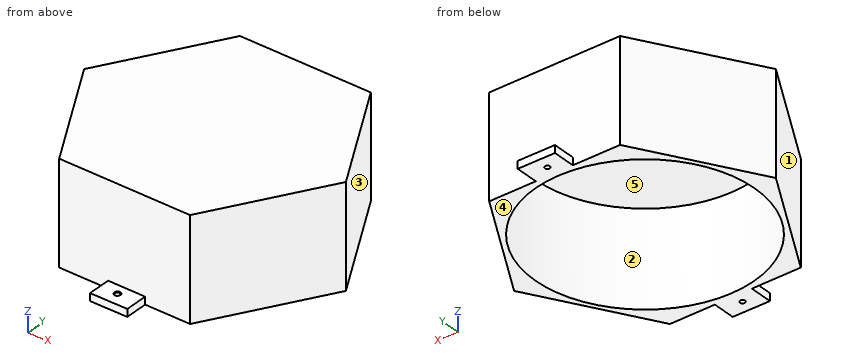
from build123d import *

# Parameters (mm, degrees)
BOSS_EXTRUDE4_DEPTH                = 40
BOSS_EXTRUDE4_DEPTH_BACK           = 1
SKETCH10_R                         = 44
CUT_EXTRUDE3_DEPTH                 = 38
SKETCH11_W                         = 15
SKETCH11_H                         = 10
BOSS_EXTRUDE5_DEPTH                = 3
M2_5X0_45_TAPPED_HOLE3_D           = 2.05
M2_5X0_45_TAPPED_HOLE3_CSINK_D     = 2.55
M2_5X0_45_TAPPED_HOLE3_CSINK_ANGLE = 90
BOSS_EXTRUDE6_DEPTH                = 41
SKETCH17_R                         = 44
CUT_EXTRUDE4_DEPTH                 = 38


with BuildPart() as part:
    # Sketch1 → Boss-Extrude4 (new body, two sides)
    with BuildSketch(Plane.XY) as boss_extrude4_sk:
        Polygon((52.078255867, 0), (26.039127933, 45.101092565), (-26.039127933, 45.101092565), (-52.078255867, 0), (-26.039127933, -45.101092565), (26.039127933, -45.101092565), align=None)
    extrude(amount=BOSS_EXTRUDE4_DEPTH)
    extrude(boss_extrude4_sk.sketch, amount=-BOSS_EXTRUDE4_DEPTH_BACK)

    # Sketch10 → Cut-Extrude3 (cut)
    with BuildSketch(Plane(origin=(0, 0, -1), x_dir=(-1, 0, 0), z_dir=(0, 0, -1))):
        Circle(SKETCH10_R)
    extrude(amount=-CUT_EXTRUDE3_DEPTH, mode=Mode.SUBTRACT)

    # Sketch11 → Boss-Extrude5 (add)
    with BuildSketch(Plane(origin=(0, 0, -1), x_dir=(-1, 0, 0), z_dir=(0, 0, -1))):
        with Locations((-0.468011799, 50.101092565)):
            Rectangle(SKETCH11_W, SKETCH11_H)
        with Locations((-0.468011799, -50.101092565)):
            Rectangle(SKETCH11_W, SKETCH11_H)
    extrude(amount=-BOSS_EXTRUDE5_DEPTH)

    # M2.5x0.45 Tapped Hole3 (through all)
    with Locations(Plane.XY.offset(2)):
        with Locations((0, 50), (0, -50)):
            CounterSinkHole(M2_5X0_45_TAPPED_HOLE3_D / 2, M2_5X0_45_TAPPED_HOLE3_CSINK_D / 2, counter_sink_angle=M2_5X0_45_TAPPED_HOLE3_CSINK_ANGLE)

    # Sketch16 → Boss-Extrude6 (add)
    with BuildSketch(Plane.XY.offset(40)):
        Polygon((-52.993622647, 0.385678178), (-26.830818423, -45.700984362), (26.162804224, -46.08666254), (52.993622647, -0.385678178), (26.830818423, 45.700984362), (-26.162804224, 46.08666254), align=None)
    extrude(amount=-BOSS_EXTRUDE6_DEPTH)

    # Sketch17 → Cut-Extrude4 (cut)
    with BuildSketch(Plane(origin=(0, 0, -1), x_dir=(-1, 0, 0), z_dir=(0, 0, -1))):
        Circle(SKETCH17_R)
    extrude(amount=-CUT_EXTRUDE4_DEPTH, mode=Mode.SUBTRACT)


solid = part.part
Design review of the part built by this model. Coordinates are the model's own, in mm. Face numbers are marked on the shaded views. A direction names the side the tool comes from. Give positions to 0.01 mm unless a question says otherwise; leave off trailing zeros. Loops run counter-clockwise (first coordinate to the right, second up) from the corner with the lowest first, then second, coordinate; pieces in that order, holes last. Notation, with made-up numbers: M 33.25,40 L 89.25,40 A28 ccw 89.25,62 Z; hole C -18.75,-29 d3. An arc over 180 degrees is marked long. One line per question, with ' | ' between items. Start each with the question number.
1. Add section C-C (x = -42). Write out the cut boundary in (y, z), plus the area to 3 significant figures.
2. To check wall thickness, follow L1, parallel to Z at x = 32.5, y = -8.5; L2, parallel to X at y = 50, z = 0 (3 decimals); L3, parallel to Y at x = -25.5, z = 4. State the ranges of each line that lie inside material, in increasing order.
3. Add section A-A (z = 14). Write out the cut boundary in (x, y), plus the area to 3 significant figures.
4. The part is to be moulded in two halves that separate along X. For the marked faces 3, 4 and 5, say which applies: released by +X, released by -X, zero draft, split by the parting line, or undercut.
5. Add section B-B (y = -10.5). Write out the cut boundary in (x, z).
6. For the marked faces 1 and 2, list the 3-axis set-ups (+Z, -Z, +X, -X, +Y, -Y) from which the entire face can be reached by the end or side of a thin tool; tool diameter is ignored.
7. Insertion check: P1, Ø3.5, axis at y = 50, z = 1, coming from the -X side; P2, Ø3, axis at x = 25.5, y = -18, coming from the -Z side; P3, Ø1, axis at y = -2.5, z = 14, coming from the +X side. Each pin has a flat end and moves straight along its axis. Give the tip position at first contact, or say it passes through.
Worked out:
1) outline: M -18.98,-1 L -13.11,-1 L -13.11,37 L 13.11,37 L 13.11,-1 L 19.11,-1 L 19.11,40 L -18.98,40 Z | area: 565 mm²
2) L1: z = 37 to 40 | L2: x = -7.032 to -1.025, 1.025 to 7.968 | L3: y = -45.71 to -35.86, 35.86 to 46.08
3) outline: M -52.99,0.39 L -26.83,-45.7 L 26.16,-46.09 L 52.99,-0.39 L 26.83,45.7 L -26.16,46.09 Z; hole C 0,0 d88 | area: 1,210 mm²
4) face 3: released by +X | face 4: zero draft | face 5: undercut
5) outline: M -46.81,-1 L -42.73,-1 L -42.73,37 L 42.73,37 L 42.73,-1 L 47.06,-1 L 47.06,40 L -46.81,40 Z
6) face 1: +Z, -Z, -X, -Y | face 2: -Z
7) P1: stops at x = -7.03 | P2: stops at z = 37 | P3: stops at x = 52.05
